from build123d import *

# Parameters (mm, degrees)
F0_W     = 87
F0_H     = 70
F0_R     = 2.5
F1_DEPTH = 7.5
F2_W     = 47
F2_H     = 60
F3_DEPTH = 5
F4_W     = 46
F4_H     = 5
F5_DEPTH = 5
F6_R     = 1
F7_R     = 2


with BuildPart() as f1:
    # F0 (on Front) → F1 (new body)
    with BuildSketch(Plane.XZ):
        with Locations((-55.98273, 20.347756)):
            Rectangle(F0_W, F0_H)
        with Locations((-94.48273, -9.152244)):
            Circle(F0_R, mode=Mode.SUBTRACT)
        with Locations((-17.48273, -9.152244)):
            Circle(F0_R, mode=Mode.SUBTRACT)
        with Locations((-94.48273, 20.347756)):
            Circle(F0_R, mode=Mode.SUBTRACT)
        with Locations((-94.48273, 49.847756)):
            Circle(F0_R, mode=Mode.SUBTRACT)
        with Locations((-17.48273, 20.347756)):
            Circle(F0_R, mode=Mode.SUBTRACT)
        with Locations((-17.48273, 49.847756)):
            Circle(F0_R, mode=Mode.SUBTRACT)
    extrude(amount=F1_DEPTH)

    # F2 (on face) → F3 (cut)
    with BuildSketch(Plane.XZ.offset(7.5)):
        with Locations((-55.98273, 20.347756)):
            Rectangle(F2_W, F2_H)
    extrude(amount=-F3_DEPTH, mode=Mode.SUBTRACT)

    # F4 (on face) → F5 (join)
    with BuildSketch(Plane.XZ.offset(7.5)):
        with Locations((-55.98273, 52.847756)):
            Rectangle(F4_W, F4_H)
        with Locations((-55.98273, -12.152244)):
            Rectangle(F4_W, F4_H)
    extrude(amount=F5_DEPTH)

    # F6
    f6_edges = [f1.edges().sort_by_distance(p)[0] for p in [
        (-78.98273, -12.5, 52.847756),
        (-32.98273, -12.5, 52.847756),
        (-32.98273, -12.5, -12.152244),
        (-78.98273, -12.5, -12.152244),
    ]]
    fillet(f6_edges, radius=F6_R)

    # F7
    f7_edges = [f1.edges().sort_by_distance(p)[0] for p in [
        (-99.48273, -3.75, -14.652244),
        (-12.48273, -3.75, -14.652244),
        (-12.48273, -3.75, 55.347756),
        (-99.48273, -3.75, 55.347756),
    ]]
    fillet(f7_edges, radius=F7_R)


solid = f1.part
Geometry: final body of the model. Coordinates: model frame, mm. A direction names the side the tool comes from. Give positions to 0.01 mm unless a question says otherwise; leave off trailing zeros. Loops run counter-clockwise (first coordinate to the right, second up) from the corner with the lowest first, then second, coordinate; pieces in that order, holes last. Notation, with made-up numbers: M 82,88 L 109,88 A25 cw 109,122 Z; hole C 29.5,19.5 d7. An arc over 180 degrees is marked long. Put each result on its own line as item: value.
1) Cut plane D-D, the plane x = -48. Return the cut outline in (y, z), plus the area to 3 significant figures.
Computed values:
outline: M -12.5,-14.65 L 0,-14.65 L 0,55.35 L -12.5,55.35 L -12.5,50.35 L -2.5,50.35 L -2.5,-9.65 L -12.5,-9.65 Z
area: 275 mm^2
2) First-contact query: P1, Ø22.5, axis at x = -92.5, z = 4, coming from the -Y side; P2, Ø2, axis at y = -10, z = 53, coming from the -X side; P3, Ø2, axis at x = -58, z = 2, coming from the -Y side. Flat tips, straight axial feed; report the tip coordinate or a pass-through.
Computed values:
P1: stops at y = -7.5
P2: stops at x = -78.98
P3: stops at y = -2.5
3) Material intervals for L1, parallel to Z at x = -44, y = -8; L2, parallel to X at y = -3.25, z = -1; L3, parallel to Z at x = -17, y = -6.75, sorted ascending. Write a range as from..to.
Computed values:
L1: z = -14.65..-9.65, 50.35..55.35
L2: x = -99.48..-79.48, -32.48..-12.48
L3: z = -14.65..-11.61, -6.7..17.89, 22.8..47.39, 52.3..55.35
4) Mould query, pull axis Z, two halves, no side actions, for faces 1 (the cylindrical face through (-16.139, -3.698, 51.956)), 2 (the flat face through (-23, -7.5, 21)), 3 (the cylindrical face through (-98.91, -3.8, 54.75)). Classes: released by +Z, released by -Z, zero draft, split by the parting line, or undercut.
Computed values:
face 1: undercut
face 2: zero draft
face 3: released by +Z
5) Cut plane C-C, the plane z = -5.5. Return the cut outline in (x, y), plus the area to 4 significant figures.
Computed values:
outline: M -99.48,-7.5 L -79.48,-7.5 L -79.48,-2.5 L -32.48,-2.5 L -32.48,-7.5 L -12.48,-7.5 L -12.48,0 L -99.48,0 Z
area: 417.5 mm^2
6) Cut plane A-A, the plane y = -9.5. Return the cut outline in (x, z).
Computed values:
outline: M -78.98,-14.65 L -32.98,-14.65 L -32.98,-9.65 L -78.98,-9.65 Z; M -78.98,50.35 L -32.98,50.35 L -32.98,55.35 L -78.98,55.35 Z
7) Reachability of faces 4 (the flat face through (-79.483, -5, 20)), 5 (the flat face through (-78.983, -9, -12)), 6 (the flat face through (-32.983, -9, 53)), 7 (the flat face through (-99.483, -4, 20)) from +Z, -Z, +X, -X, +Y, -Y: full face, straight path, thin tool, end or side. Return the list, or none.
Computed values:
face 4: -Y
face 5: +Z, -Z, -X, -Y
face 6: +Z, -Z, +X, -Y
face 7: +Z, -Z, -X, +Y, -Y
8) Cut plane B-B, the plane x = -93. Return the cut outline in (y, z), plus the area to 3 significant figures.
Computed values:
outline: M -7.5,-14.65 L 0,-14.65 L 0,-11.17 L -7.5,-11.17 Z; M -7.5,-7.14 L 0,-7.14 L 0,18.33 L -7.5,18.33 Z; M -7.5,22.36 L 0,22.36 L 0,47.83 L -7.5,47.83 Z; M -7.5,51.86 L 0,51.86 L 0,55.35 L -7.5,55.35 Z
area: 434 mm^2
